Model file for the job. Use its own axes, mm. Give positions to 0.01 mm unless a question says otherwise; leave off trailing zeros. Write each loop counter-clockwise with the first axis right and the second up, starting at its lowest first coordinate (ties: lowest second). Pieces come first, ordered by that corner, then holes. Notation, with made-up numbers: (32.5, 5) - (85.5, 5) arc R14 ccw to (85.5, 9) - close; hole circle Ø6 at (-5.75, -36.5). An arc over 180 degrees is marked (long way). One line per item, written item: value. Start each with the question number.
(1) Drop a flat-ended pin along its axis: P1, Ø1, axis at x = 28, y = 120, coming from the -Z side. Give the stop position or say it passes through.
(2) Cut at B-B, the plane y = -280. List the corners of the cut face in (x, z), and give its area (3 significant figures).
(3) Probe L1, parallel to Y at x = 0, z = 2.8; L2, parallel to X at y = 0, z = 2.7; L3, parallel to Y at x = 1.5, z = 3. List the from-to ranges inside material, lowest first.
(4) Cut at A-A, the plane x = 0. List the corners of the cut face in (y, z), and give its area (3 significant figures).
from build123d import *

# Parameters (mm, degrees)
F0_W     = 80
F0_H     = 600
F1_DEPTH = 5
F2_R     = 6
F3_DEPTH = 25


with BuildPart() as f1:
    # F0 (on Top) → F1 (new body)
    with BuildSketch(Plane.XY):
        Rectangle(F0_W, F0_H)
    extrude(amount=F1_DEPTH)

    # F2 (on Top) → F3 (cut)
    with BuildSketch(Plane.XY):
        with Locations((0, 280)):
            Circle(F2_R)
        Circle(F2_R)
        with Locations((0, -280)):
            Circle(F2_R)
    extrude(amount=F3_DEPTH, mode=Mode.SUBTRACT)


solid = f1.part
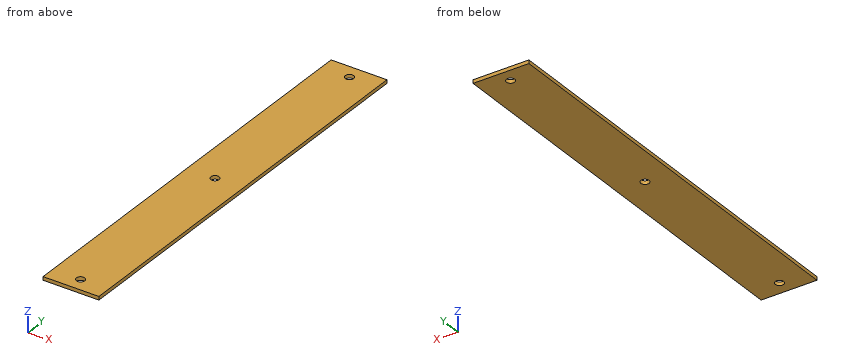
Answers follow:
1. P1: stops at z = 0
2. outline: (-40, 0) - (-6, 0) - (-6, 5) - (-40, 5) - close; (6, 0) - (40, 0) - (40, 5) - (6, 5) - close
2. area: 340 mm²
3. L1: y = -300 to -286, -274 to -6, 6 to 274, 286 to 300
3. L2: x = -40 to -6, 6 to 40
3. L3: y = -300 to -285.81, -274.19 to -5.81, 5.81 to 274.19, 285.81 to 300
4. outline: (-300, 0) - (-286, 0) - (-286, 5) - (-300, 5) - close; (-274, 0) - (-6, 0) - (-6, 5) - (-274, 5) - close; (6, 0) - (274, 0) - (274, 5) - (6, 5) - close; (286, 0) - (300, 0) - (300, 5) - (286, 5) - close
4. area: 2,820 mm²
